Check sheet for the modelled part. Datum: model origin and axes. Units: mm. A direction names the side the tool comes from. Round coordinates to 2 decimals unless told otherwise and drop trailing zeros. Order: outer loops, then holes, each group sorted by start corner. A loop starts at its lowest first (then second) coordinate and runs counter-clockwise, first axis right, second up. Notation, with made-up numbers: (-35, 9.5) -> (-14, 9.5) arc R19 ccw to (-14, 18.5) -> close; hole circle Ø10 at (81.25, -16.75). An arc over 180 degrees is marked (long way). Answer in a Markdown table with one row per item.
from build123d import *

# Parameters (mm, degrees)
BOSS_EXTRUDE1_DEPTH    = 18
SKETCH1_3_R            = 7
BOSS_EXTRUDE2_DEPTH    = 12
SKETCH2_R              = 12
BOSS_EXTRUDE3_DEPTH    = 4.5
RIB1_REACH             = 77.186
SKETCH3_WALL_W         = 190.924782946
SKETCH3_WALL_H         = 6
F_12_0MM_DOWEL_HOLE1_D = 12


with BuildPart() as part:
    # Sketch1 → Boss-Extrude1 (new, symmetric)
    with BuildSketch(Plane.XY):
        with BuildLine():
            Line((55, 5), (23.473389189, 5))
            ThreePointArc((23.473389189, 5), (23.86798421, 2.513827706), (24, 0))
            Line((24, 0), (55, 0))
            Line((55, 0), (55, 5))
        make_face()
        with BuildLine():
            ThreePointArc((0, 24), (-16.970562748, 16.970562748), (-24, 0))
            Line((-24, 0), (-18, 0))
            ThreePointArc((-18, 0), (0, 18), (18, 0))
            Line((18, 0), (24, 0))
            ThreePointArc((24, 0), (23.86798421, 2.513827706), (23.473389189, 5))
            ThreePointArc((23.473389189, 5), (15.099668871, 18.654758106), (0, 24))
        make_face()
    extrude(amount=BOSS_EXTRUDE1_DEPTH, both=True)

    # Sketch1_3 → Boss-Extrude2 (add, symmetric)
    with BuildSketch(Plane.XY):
        with BuildLine():
            Line((-24, 36), (-24, 0))
            ThreePointArc((-24, 0), (-16.970562748, 16.970562748), (0, 24))
            Line((0, 24), (0, 36))
            ThreePointArc((0, 36), (-12, 48), (-24, 36))
        make_face()
        with Locations((-12, 36)):
            Circle(SKETCH1_3_R, mode=Mode.SUBTRACT)
    extrude(amount=BOSS_EXTRUDE2_DEPTH, both=True)

    # Sketch2 → Boss-Extrude3 (add, symmetric)
    with BuildSketch(Plane(origin=(0, 5, 0), x_dir=(1, 0, 0), z_dir=(0, 1, 0))):
        with Locations((40, 0)):
            Circle(SKETCH2_R)
    extrude(amount=BOSS_EXTRUDE3_DEPTH, both=True)

    # Sketch3 wall → Rib1 (add, up to next)
    with BuildSketch(Plane(origin=(14, 22.75, 0), x_dir=(0.72629339981, -0.68738482482, 0), z_dir=(0.68738482482, 0.72629339981, 0)), mode=Mode.PRIVATE) as rib1_sk1:
        Rectangle(SKETCH3_WALL_W, SKETCH3_WALL_H)
    rib1_tool1 = extrude(rib1_sk1.sketch, amount=-RIB1_REACH, mode=Mode.PRIVATE) - part.part
    add(rib1_tool1.solids().sort_by_distance((14, 22.75, 0))[0])

    # 12.0mm Dowel Hole1 (through all)
    with Locations(Plane(origin=(0, 9.5, 0), x_dir=(1, 0, 0), z_dir=(0, 1, 0))):
        with Locations((40, 0)):
            Hole(F_12_0MM_DOWEL_HOLE1_D / 2)


solid = part.part
Item 1: Cross-section at B-B (y = 4). Record the boundary of the cut face in (x, z).
Result sheet:
| item | result |
|---|---|
| outline | (-24, -12) -> (-23.66, -12) -> (-23.66, -18) -> (-17.55, -18) -> (-17.55, 18) -> (-23.66, 18) -> (-23.66, 12) -> (-24, 12) -> close; (17.55, -18) -> (55, -18) -> (55, 18) -> (17.55, 18) -> close; hole circle Ø12 at (40, 0) |
Item 2: Scan lines: line 1 (Z direction, x = 40, y = 3); line 2 (Y direction, x = 39.5, z = -14); line 3 (Y direction, x = -12, z = 7). Record each from-to range of solid material in increasing order. Write a range as [from, to].
Result sheet:
| item | result |
|---|---|
| line 1 | z = [-18, -6], [6, 18] |
| line 2 | y = [0, 5] |
| line 3 | y = [13.42, 29], [43, 48] |
Item 3: Cross-section at A-A (x = 40). Record the boundary of the cut face in (y, z).
Result sheet:
| item | result |
|---|---|
| outline | (0, -18) -> (5, -18) -> (5, -12) -> (9.5, -12) -> (9.5, -6) -> (0, -6) -> close; (0, 6) -> (9.5, 6) -> (9.5, 12) -> (5, 12) -> (5, 18) -> (0, 18) -> close |
Item 4: Set-up check for faces 1 (the flat face through (42, 9.5, -6)), 2 (the flat face through (0, 30, -7)), 3 (the flat face through (39.5, 5, 12.3)), 4 (the flat face through (13.4, 20.1, 3)), 5 (the cylindrical face through (5.736, 23.304, -12.062)): record each of +Z, -Z, +X, -X, +Y, -Y from which the full face is reachable in a straight line by a thin tool's end or side.
Result sheet:
| item | result |
|---|---|
| face 1 | +Z, -Z, +X, +Y |
| face 2 | -Z, +X, +Y |
| face 3 | +Y |
| face 4 | +Z, +Y |
| face 5 | -Z, +Y |
Item 5: Mould release check, pull along Z, two halves, no side actions. Record for faces 6 (the cylindrical face through (46, 5, 0)), 7 (the flat face through (15.3, 10.3, 18)), 8 (the cylindrical face through (0, 18, 0)), 9 (the flat face through (13.4, 20.1, -3)): pulls with the +Z half, pulls with the -Z half, needs draft (parallel to the pull), parting line crosses it, or undercut.
Result sheet:
| item | result |
|---|---|
| face 6 | undercut |
| face 7 | pulls with the +Z half |
| face 8 | needs draft |
| face 9 | pulls with the -Z half |
Item 6: Cross-section at D-D (z = 15.5). Record the boundary of the cut face in (x, y), and give its area (3 significant figures).
Result sheet:
| item | result |
|---|---|
| outline | (-24, 0) -> (-18, 0) arc R18 cw to (18, 0) -> (55, 0) -> (55, 5) -> (23.47, 5) arc R24 ccw to start |
| area | 552 mm^2 |
Item 7: Depth check by flat-ended pin: P1, Ø10, axis at y = 28, z = -6, coming from the +X side; P2, Ø4, axis at y = 22, z = -10, coming from the +X side; P3, Ø10, axis at x = 33.5, z = -3, coming from the +Y side. Enter the tip coordinate at first touch or a pass-through.
Result sheet:
| item | result |
|---|---|
| P1 | stops at x = 12.68 |
| P2 | stops at x = 13.27 |
| P3 | stops at y = 9.5 |
Item 8: Cross-section at C-C (y = 42). Record the boundary of the cut face in (x, z), and give its area (3 significant figures).
Result sheet:
| item | result |
|---|---|
| outline | (-22.39, -12) -> (-15.61, -12) -> (-15.61, 12) -> (-22.39, 12) -> close; (-8.39, -12) -> (-1.61, -12) -> (-1.61, 12) -> (-8.39, 12) -> close |
| area | 326 mm^2 |
